Build history of the part. All positions in model axes, mm. Face numbers are marked on the shaded views. A direction names the side the tool comes from. Round coordinates to 2 decimals unless told otherwise and drop trailing zeros. Write each loop counter-clockwise with the first axis right and the second up, starting at its lowest first coordinate (ties: lowest second). Pieces come first, ordered by that corner, then holes.
from build123d import *

# Parameters (mm, degrees)
CROQUIS1_R                    = 140
SALIENTE_EXTRUIR1_DEPTH       = 3
SALIENTE_EXTRUIR2_DEPTH       = 35
CROQUIS3_5_R                  = 30
CROQUIS3_5_R_2                = 13.2
CORTAR_EXTRUIR3_DEPTH         = 150
TALADRO_DE_MARGEN_PARA_3_81_D = 10.0838
CORTAR_EXTRUIR4_DEPTH         = 10
REDONDEO1_R                   = 20
CROQUIS7_R                    = 15
CORTAR_EXTRUIR5_DEPTH         = 3
ESCALA1_SCALE                 = 1.15


with BuildPart() as part:
    # Croquis1 → Saliente-Extruir1 (new body)
    with BuildSketch(Plane(origin=(0, 0, 0), x_dir=(1, 0, 0), z_dir=(0, 1, 0))):
        with Locations(Location((0, 0, 0), (0, 0, 270))):
            Circle(CROQUIS1_R)
    extrude(amount=SALIENTE_EXTRUIR1_DEPTH)

    # Croquis3 → Saliente-Extruir2 (add)
    with BuildSketch(Plane(origin=(0, 0, 0), x_dir=(-1, 0, 0), z_dir=(0, -1, 0))):
        with BuildLine():
            Line((2.5, -102.46950766), (-2.5, -102.46950766))
            Line((-2.5, -102.46950766), (-2.5, -43.928919859))
            ThreePointArc((-2.5, -43.928919859), (-14.696982207, -19.344018802), (-41.651497534, -14.182833045))
            Line((-41.651497534, -14.182833045), (-98.050103968, -29.873518571))
            Line((-98.050103968, -29.873518571), (-99.390258391, -25.056466971))
            Line((-99.390258391, -25.056466971), (-42.991651956, -9.365781444))
            ThreePointArc((-42.991651956, -9.365781444), (-11.672149328, -15.36276447), (2.5, -43.928919859))
            Line((2.5, -43.928919859), (2.5, -102.46950766))
        make_face()
    extrude(amount=-SALIENTE_EXTRUIR2_DEPTH)

    # Croquis3<5> → Cortar-Extruir3 (cut)
    with BuildSketch(Plane(origin=(0, 0, 0), x_dir=(-1, 0, 0), z_dir=(0, -1, 0))):
        Polygon((12.227859388, -30.111948705), (30.38932597, -97.89146473), (102.481249664, -1.960476316), (32.393429517, -2.62977644), align=None)
        with Locations(Location((-36.766027199, -50.10571417, 0), (0, 0, 90))):
            Circle(CROQUIS3_5_R)
        Polygon((-30.38932597, 97.89146473), (-102.481249664, 1.960476316), (-32.393429517, 2.62977644), (-12.227859388, 30.111948705), align=None)
        with BuildLine():
            Line((30.547985144, 11.093719108), (98.050103968, 29.873518571))
            Line((98.050103968, 29.873518571), (2.5, 102.46950766))
            Line((2.5, 102.46950766), (2.5, 32.403703492))
            ThreePointArc((2.5, 32.403703492), (19.661413711, 25.878153158), (30.547985144, 11.093719108))
        make_face()
        with Locations(Location((0, 0, 0), (0, 0, 90))):
            Circle(CROQUIS3_5_R_2)
    extrude(amount=-CORTAR_EXTRUIR3_DEPTH, mode=Mode.SUBTRACT)

    # Taladro de margen para 3/81 (through all)
    with Locations(Plane(origin=(0, 3, 0), x_dir=(1, 0, 0), z_dir=(0, 1, 0))):
        with Locations((58.047355757, -109.461018128), (89.897390413, -85.262355099), (-58.047355757, 109.461018128), (-89.897390413, 85.262355099)):
            Hole(TALADRO_DE_MARGEN_PARA_3_81_D / 2)

    # Croquis6 → Cortar-Extruir4 (cut)
    with BuildSketch(Plane(origin=(0, 3, 0), x_dir=(1, 0, 0), z_dir=(0, 1, 0))):
        with BuildLine():
            Line((-92.55315644, 47.433250289), (-138.14042031, 107.434744271))
            ThreePointArc((-138.14042031, 107.434744271), (-139.34390162, -105.869150753), (66.477842334, -161.881736087))
            Line((66.477842334, -161.881736087), (20.890578464, -101.880242105))
            ThreePointArc((20.890578464, -101.880242105), (-82.810090106, -62.916523876), (-92.55315644, 47.433250289))
        make_face()
        with BuildLine():
            Line((-66.477842334, 161.881736087), (-20.890578464, 101.880242105))
            ThreePointArc((-20.890578464, 101.880242105), (82.810090106, 62.916523876), (92.55315644, -47.433250289))
            Line((92.55315644, -47.433250289), (138.14042031, -107.434744271))
            ThreePointArc((138.14042031, -107.434744271), (139.34390162, 105.869150753), (-66.477842334, 161.881736087))
        make_face()
    extrude(amount=-CORTAR_EXTRUIR4_DEPTH, mode=Mode.SUBTRACT)

    # Redondeo1
    redondeo1_edges = [part.edges().sort_by_distance(p)[0] for p in [
        (-30.547985144, 1.5, -11.093719108),
        (-2.5, 1.5, -32.403703492),
        (-2.5, 1.5, -102.46950766),
        (-98.050103968, 1.5, -29.873518571),
        (-12.227859388, 1.5, 30.111948705),
        (-32.393429517, 1.5, 2.62977644),
        (-102.481249664, 1.5, 1.960476316),
        (-30.38932597, 1.5, 97.89146473),
        (12.227859388, 1.5, -30.111948705),
        (32.393429517, 1.5, -2.62977644),
        (102.481249664, 1.5, -1.960476316),
        (30.38932597, 1.5, -97.89146473),
    ]]
    fillet(redondeo1_edges, radius=REDONDEO1_R)

    # Croquis7 → Cortar-Extruir5 (cut)
    with BuildSketch(Plane.XZ):
        with Locations(Location((0, 0, 0), (0, 0, 270))):
            Circle(CROQUIS7_R)
    extrude(amount=-CORTAR_EXTRUIR5_DEPTH, mode=Mode.SUBTRACT)


with BuildPart() as part_1:
    # Escala1: scaled about (8.077452508, 6.145488529, 10.496326588)
    add(part.part.scale(ESCALA1_SCALE).moved(Location((-1.211617876, -0.921823279, -1.574448988))))


solid = part_1.part
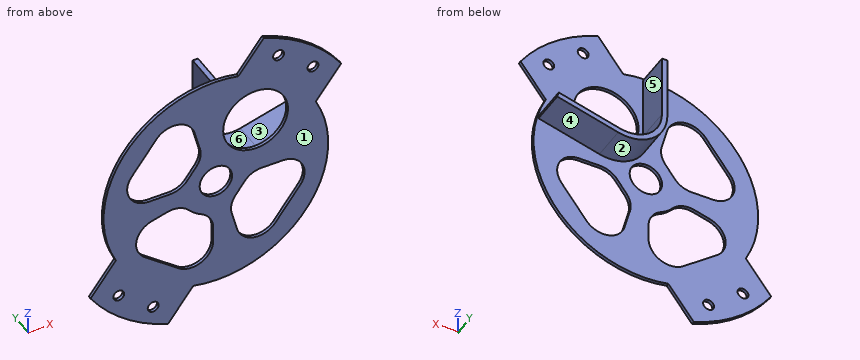
1) Wall check: L1, parallel to Y at x = 90, z = 83; L2, parallel to X at y = 17, z = 48; L3, parallel to Z at x = 37.5, y = 10. Give the ranges that are in metal, low to high.
Results:
L1: y = -0.92 to 2.53
L2: x = -4.08 to 1.68
L3: z = 7.69 to 13.44
2) Slice it at A-A (x = 34). Write the cut outline in (y, z).
Results:
outline: (-0.92, -115.87) - (2.53, -115.87) - (2.53, -83.41) - (-0.92, -83.41) - close; (-0.92, -9.07) - (2.53, -9.07) - (2.53, 7.81) - (39.33, 7.81) - (39.33, 13.58) - (2.53, 13.58) - (2.53, 22.28) - (-0.92, 22.28) - close; (-0.92, 89.82) - (2.53, 89.82) - (2.53, 130.31) - (-0.92, 130.31) - close
3) Mould opens along X. For the marked faces 1, 2, 3 and 4 say: released by +X, released by -X, zero draft, split by the parting line, or undercut.
Results:
face 1: zero draft
face 2: split by the parting line
face 3: undercut
face 4: released by +X
4) Which spindle directions (+Z, -Z, +X, -X, +Y, -Y) get a long thin tool onto all of the face, cutting with end or side? Do the marked faces 5 and 6. Say none if no direction does.
Results:
face 5: +Z, +X, +Y
face 6: +Z, +Y
5) Slice it at D-D (x = -12). Write the cut outline in (y, z), plus the area to 3 significant figures.
Results:
outline: (-0.92, -120.69) - (2.53, -120.69) - (2.53, -90.42) - (-0.92, -90.42) - close; (-0.92, -38.76) - (2.53, -38.76) - (2.53, -15.03) - (-0.92, -15.03) - close; (-0.92, 11.89) - (2.53, 11.89) - (2.53, 117.54) - (-0.92, 117.54) - close
area: 551 mm2
6) Pin check, flat tips, straight feed: pin 1 Ø4.5 at (x, y) = (-1.5, 22) entering from +Z; pin 2 Ø4 at (y, z) = (0.5, -68) entering from -X; pin 3 Ø10 at (x, y) = (-91, 6.5) entering from +Z. Stop position of each tip, or through.
Results:
pin 1: stops at z = 116.27
pin 2: stops at x = -118.19
pin 3: stops at z = 80.76
7) Slice it at C-C (z = 110.5). Write the cut outline in (x, y).
Results:
outline: (-42.97, -0.92) - (114.38, -0.92) - (114.38, 2.53) - (1.66, 2.53) - (1.66, 39.33) - (-4.09, 39.33) - (-4.09, 2.53) - (-42.97, 2.53) - close
8) Slice it at B-B (y = 18.5). Write the cut outline in (x, z), plus the area to 3 significant figures.
Results:
outline: (-4.09, 48.94) arc R41.26 ccw to (48.23, 9.2) - (113.09, 27.24) - (111.55, 32.78) - (46.69, 14.74) arc R35.51 cw to (1.66, 48.94) - (1.66, 116.27) - (-4.09, 116.27) - close
area: 1,180 mm2
